from build123d import *

# Parameters (mm, degrees)
SKETCH020_W             = 431.8
SKETCH020_H             = 279.4
PAD001_DEPTH            = 1.5748
SKETCH017_R             = 2.61
POCKET019_DEPTH         = 5
LINEARPATTERN014_COUNT  = 4
LINEARPATTERN014_PITCH  = 50
LINEARPATTERN009_COUNT  = 4
LINEARPATTERN009_PITCH  = 50
SKETCH012_R             = 2.61
POCKET015_DEPTH         = 1.5758
LINEARPATTERN008_COUNT  = 3
LINEARPATTERN008_PITCH  = 50
LINEARPATTERN013_COUNT  = 3
LINEARPATTERN013_PITCH  = 50
SKETCH015_R             = 2.61
POCKET016_DEPTH         = 1.5758
LINEARPATTERN010_COUNT  = 4
LINEARPATTERN010_PITCH  = 50
LINEARPATTERN011_COUNT  = 4
LINEARPATTERN011_PITCH  = 50
SKETCH018_R             = 2.61
POCKET018_DEPTH         = 1.5758
LINEARPATTERN015_COUNT  = 3
LINEARPATTERN015_PITCH  = 50
LINEARPATTERN012_COUNT  = 3
LINEARPATTERN012_PITCH  = 50
SKETCH019_R             = 2.95
POCKET017_DEPTH         = 1.5758
BODY001_PLACEMENT_ANGLE = 90


with BuildPart() as part:
    # Sketch020 → Pad001 (new body)
    with BuildSketch(Plane.XY):
        with Locations((0, 139.7)):
            Rectangle(SKETCH020_W, SKETCH020_H)
    extrude(amount=PAD001_DEPTH)

    # Sketch017 → Pocket019 (cut)
    with BuildSketch(Plane.XY):
        with Locations((0, 9)):
            Circle(SKETCH017_R)
    pocket019 = extrude(amount=POCKET019_DEPTH, mode=Mode.SUBTRACT)

    # LinearPattern014: Pocket019 ×4
    with Locations(*[(i * LINEARPATTERN014_PITCH, 0, 0) for i in range(1, LINEARPATTERN014_COUNT)]):
        add(pocket019, mode=Mode.SUBTRACT)

    # LinearPattern009: Pocket019 ×4
    with Locations(*[(-i * LINEARPATTERN009_PITCH, 0, 0) for i in range(1, LINEARPATTERN009_COUNT)]):
        add(pocket019, mode=Mode.SUBTRACT)

    # Sketch012 → Pocket015 (cut, through all)
    with BuildSketch(Plane.XY):
        with Locations((-206.9, 130.7)):
            Circle(SKETCH012_R)
    pocket015 = extrude(amount=POCKET015_DEPTH, mode=Mode.SUBTRACT)

    # LinearPattern008: Pocket015 ×3
    with Locations(*[(0, -i * LINEARPATTERN008_PITCH, 0) for i in range(1, LINEARPATTERN008_COUNT)]):
        add(pocket015, mode=Mode.SUBTRACT)

    # LinearPattern013: Pocket015 ×3
    with Locations(*[(0, i * LINEARPATTERN013_PITCH, 0) for i in range(1, LINEARPATTERN013_COUNT)]):
        add(pocket015, mode=Mode.SUBTRACT)

    # Sketch015 → Pocket016 (cut, through all)
    with BuildSketch(Plane.XY):
        with Locations((0, 270.4)):
            Circle(SKETCH015_R)
    pocket016 = extrude(amount=POCKET016_DEPTH, mode=Mode.SUBTRACT)

    # LinearPattern010: Pocket016 ×4
    with Locations(*[(i * LINEARPATTERN010_PITCH, 0, 0) for i in range(1, LINEARPATTERN010_COUNT)]):
        add(pocket016, mode=Mode.SUBTRACT)

    # LinearPattern011: Pocket016 ×4
    with Locations(*[(-i * LINEARPATTERN011_PITCH, 0, 0) for i in range(1, LINEARPATTERN011_COUNT)]):
        add(pocket016, mode=Mode.SUBTRACT)

    # Sketch018 → Pocket018 (cut, through all)
    with BuildSketch(Plane.XY):
        with Locations((206.9, 130.7)):
            Circle(SKETCH018_R)
    pocket018 = extrude(amount=POCKET018_DEPTH, mode=Mode.SUBTRACT)

    # LinearPattern015: Pocket018 ×3
    with Locations(*[(0, i * LINEARPATTERN015_PITCH, 0) for i in range(1, LINEARPATTERN015_COUNT)]):
        add(pocket018, mode=Mode.SUBTRACT)

    # LinearPattern012: Pocket018 ×3
    with Locations(*[(0, -i * LINEARPATTERN012_PITCH, 0) for i in range(1, LINEARPATTERN012_COUNT)]):
        add(pocket018, mode=Mode.SUBTRACT)

    # Sketch019 → Pocket017 (cut, through all)
    with BuildSketch(Plane.XY):
        with Locations((-177.8, 177.8)):
            Circle(SKETCH019_R)
        with Locations((-177.8, 25.4)):
            Circle(SKETCH019_R)
    extrude(amount=POCKET017_DEPTH, mode=Mode.SUBTRACT)


with BuildPart() as part_1:
    # Body001 placement: moved
    add(part.part.moved(Location((-81, -61, -198))).rotate(Axis((-81, -61, -198), (-1, 0, 0)), BODY001_PLACEMENT_ANGLE))


solid = part_1.part
Geometry check sheet. Reference: the model listing, model coordinates, mm. Coordinates: 2 decimals unless noted, no trailing zeros. Answer in a Markdown table with one row per item. Add a question column.
1) Gauge pin test, flat end, axial feed: P1, Ø4.5, axis at x = 125.9, z = -228.7, coming from the +Y side. Record the tip position at first contact, or that the pin passes through.
2) Release check for a two-part mould opening along Y. For faces 1 (the flat face through (-84, -61, -340)), 2 (the flat face through (-84, -59.425, -340)) record: +Y half, -Y half, draft (parallel to the pull), parting line (faces both ways), or undercut.
3) Material ranges on line 1 along Z through (x, y) = (-31, -60.5); line 2 along Z through (x, y) = (-287.9, -60.25); line 3 along X through (y, z) = (-60, -375.8), recorded low to high. Write a range as [from, to].
Check result:
| question | item | result |
|---|---|---|
| 1 | P1 | passes through |
| 2 | face 1 | -Y half |
| 2 | face 2 | +Y half |
| 3 | line 1 | z = [-477.4, -471.01], [-465.79, -209.61], [-204.39, -198] |
| 3 | line 2 | z = [-477.4, -431.31], [-426.09, -381.31], [-376.09, -331.31], [-326.09, -281.31], [-276.09, -231.31], [-226.09, -198] |
| 3 | line 3 | x = [-296.9, -261.75], [-255.85, 134.9] |
